Answer from the drawing. Dimensions are ordinates in mm from the lowest x, y and z of the part. A direction names the side the tool comes from. Give positions to 0.01 mm unless a question says otherwise; leave off trailing zeros. Loops run counter-clockwise (first coordinate to the right, second up) from the corner with the lowest first, then second, coordinate; pieces in that order, holes last.
(1) Which of the six approach directions +Z, -Z, +X, -X, +Y, -Y give full straight-line access (tool end or side, diameter ignored) to the marked faces 1, 2 and 3?
(2) Find section A-A, the plane y = 4. Write down the section's boundary in (x, z), then the cut area to 3 significant figures.
(3) Determine the mould class of the marked faces 4, 5 and 6 for opening direction X: pulls with the +X half, pulls with the -X half, needs draft (parallel to the pull), parting line crosses it, or undercut.
(4) Find section B-B, the plane z = 1.35. Write down the section's boundary in (x, y).
(5) This flat-tipped pin is pushed along its axis until it touches: P1, Ø2, axis at y = 5.5, z = 1.5, coming from the -X side. Where does it stop, or does it pass through?
(6) Straight lines are drawn through the part: probe 1 along Y at (x, z) = (3.5, 3); probe 2 along X at (y, z) = (2.75, 2.4); probe 3 along Z at (x, y) = (6.75, 5). For each, find the intervals that lie inside material, in ascending order.
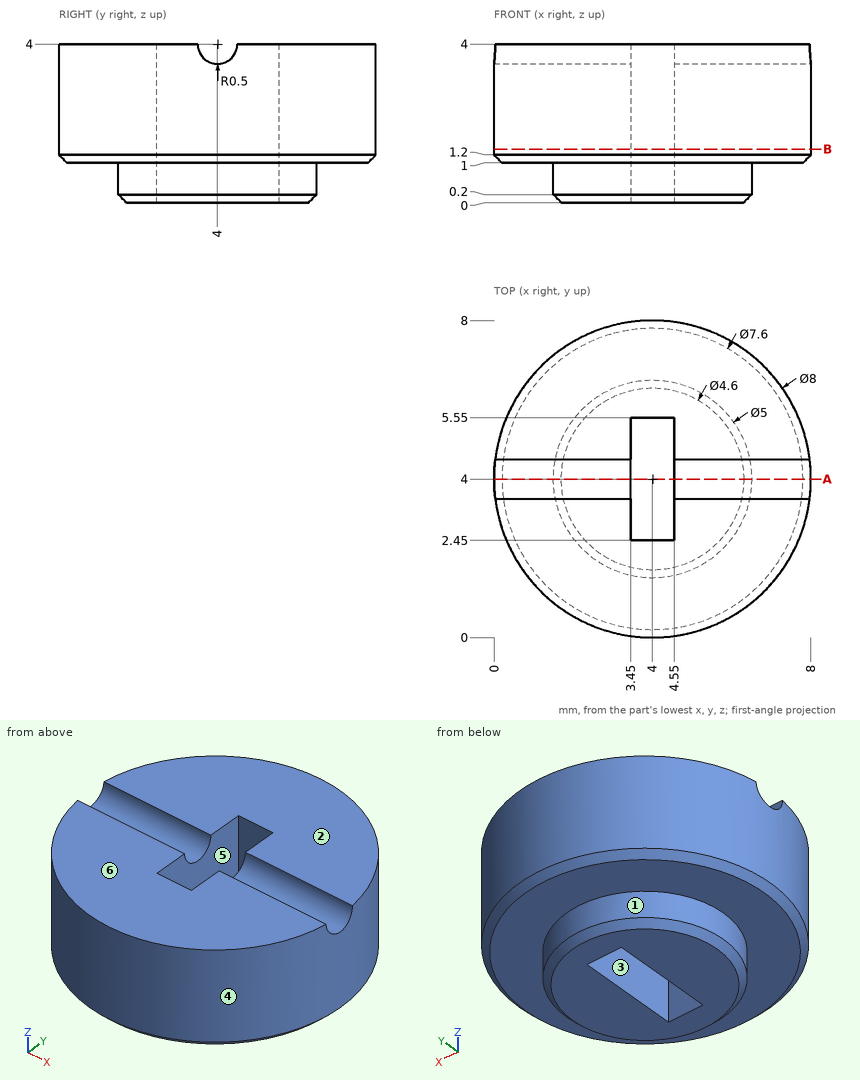
Entries:
1. face 1: -Z
1. face 2: +Z, +X, -X, +Y, -Y
1. face 3: +Z, -Z
2. outline: (0, 1.2) - (0.2, 1) - (1.5, 1) - (1.5, 0.2) - (1.7, 0) - (3.45, 0) - (3.45, 3.5) - (0, 3.5) - close; (4.55, 0) - (6.3, 0) - (6.5, 0.2) - (6.5, 1) - (7.8, 1) - (8, 1.2) - (8, 3.5) - (4.55, 3.5) - close
2. area: 21.1 mm2
3. face 4: parting line crosses it
3. face 5: undercut
3. face 6: needs draft
4. outline: circle Ø8 at (4, 4); hole (3.45, 2.45) - (4.55, 2.45) - (4.55, 5.55) - (3.45, 5.55) - close
5. P1: stops at x = 0.03
6. probe 1: y = 0.03 to 2.45, 5.55 to 7.97
6. probe 2: x = 0.2 to 3.45, 4.55 to 7.8
6. probe 3: z = 1 to 4
